Source: CAD feature listing. Evaluate the final solid. Frame: model axes, mm. A direction names the side the tool comes from. Coordinates: 2 decimals unless noted, no trailing zeros. Loops run counter-clockwise (first coordinate to the right, second up) from the corner with the lowest first, then second, coordinate; pieces in that order, holes last. Notation, with made-up numbers: (53, 36.25) -> (101, 36.25) arc R3 cw to (101, 40.25) -> close; hole circle Ø9 at (9, -34.5). An arc over 180 degrees is marked (long way). Answer as a JSON object with one key per item and string values. Group by question number.
from build123d import *

# Parameters (mm, degrees)
SKETCH1_R           = 4
BOSS_EXTRUDE1_DEPTH = 8
SKETCH2_R           = 10
BOSS_EXTRUDE2_DEPTH = 26
SKETCH3_R           = 12.5
BOSS_EXTRUDE3_DEPTH = 38
SKETCH4_R           = 10
BOSS_EXTRUDE4_DEPTH = 20
SKETCH5_R           = 7.5
BOSS_EXTRUDE5_DEPTH = 34
SKETCH8_R           = 10
SKETCH8_R_2         = 7.5
BOSS_EXTRUDE6_DEPTH = 7


with BuildPart() as part:
    # Sketch1 → Boss-Extrude1 (new body)
    with BuildSketch(Plane.XY):
        Circle(SKETCH1_R)
    extrude(amount=BOSS_EXTRUDE1_DEPTH)

    # Sketch2 → Boss-Extrude2 (add)
    with BuildSketch(Plane.XY.offset(8)):
        with Locations(Location((0, 0, 0), (0, 0, 180))):
            Circle(SKETCH2_R)
    extrude(amount=BOSS_EXTRUDE2_DEPTH)

    # Sketch3 → Boss-Extrude3 (add)
    with BuildSketch(Plane.XY.offset(34)):
        Circle(SKETCH3_R)
    extrude(amount=BOSS_EXTRUDE3_DEPTH)

    # Sketch4 → Boss-Extrude4 (add)
    with BuildSketch(Plane.XY.offset(72)):
        with Locations(Location((0, 0, 0), (0, 0, 180))):
            Circle(SKETCH4_R)
    extrude(amount=BOSS_EXTRUDE4_DEPTH)

    # Sketch5 → Boss-Extrude5 (add)
    with BuildSketch(Plane.XY.offset(92)):
        Circle(SKETCH5_R)
    extrude(amount=BOSS_EXTRUDE5_DEPTH)

    # Sketch8 → Boss-Extrude6 (add)
    with BuildSketch(Plane.XY.offset(92)):
        with Locations(Location((0, 0, 0), (0, 0, 180))):
            Circle(SKETCH8_R)
        Circle(SKETCH8_R_2, mode=Mode.SUBTRACT)
    extrude(amount=BOSS_EXTRUDE6_DEPTH)


solid = part.part
1. Pin query (flat end, axial travel): pin 1 Ø4 at (y, z) = (-6.5, 28.5) entering from +X; pin 2 Ø1.5 at (y, z) = (2, 33) entering from -X; pin 3 Ø2 at (x, y) = (-8, 4.5) entering from -Z. Return the tip coordinate at first contact, or that it passes through.
2. Section query C-C on z = 42. Return loops of the section in (x, y).
3. Section query A-A on x = 0. Return loops of the section in (y, z).
4. Ray query, L1, parallel to Z at x = -4.25, y = -8.25; L2, parallel to Z at x = -10.25, y = 6.5; L3, parallel to X at y = 10, z = 58. Return the intervals inside material, ascending.
5. Section query D-D on x = -5.5. Return loops of the section in (y, z), then the cut area to 3 significant figures.
6. Reachability of faces 1 (the face through (-0.1, 10.2, 34)), 2 (the face through (11.923, 3.755, 52.734)), 3 (the face through (10, 0, 85)) from +Z, -Z, +X, -X, +Y, -Y: full face, straight path, thin tool, end or side. Return the list, or none.
Solved:
{
 "1": {"pin 1": "x = 8.93", "pin 2": "x = -9.92", "pin 3": "z = 8"},
 "2": {"outline": "circle Ø25 at (0, 0)"},
 "3": {"outline": "(-12.5, 34) -> (-10, 34) -> (-10, 8) -> (-4, 8) -> (-4, 0) -> (4, 0) -> (4, 8) -> (10, 8) -> (10, 34) -> (12.5, 34) -> (12.5, 72) -> (10, 72) -> (10, 99) -> (7.5, 99) -> (7.5, 126) -> (-7.5, 126) -> (-7.5, 99) -> (-10, 99) -> (-10, 72) -> (-12.5, 72) -> close"},
 "4": {"L1": "8 to 99", "L2": "34 to 72", "L3": "-7.5 to 7.5"},
 "5": {"outline": "(-11.22, 34) -> (-8.35, 34) -> (-8.35, 8) -> (8.35, 8) -> (8.35, 34) -> (11.22, 34) -> (11.22, 72) -> (8.35, 72) -> (8.35, 99) -> (5.1, 99) -> (5.1, 126) -> (-5.1, 126) -> (-5.1, 99) -> (-8.35, 99) -> (-8.35, 72) -> (-11.22, 72) -> close", "area": "2,010 mm^2"},
 "6": {"face 1": "-Z", "face 2": "+Z, -Z", "face 3": "+Z"}
}
